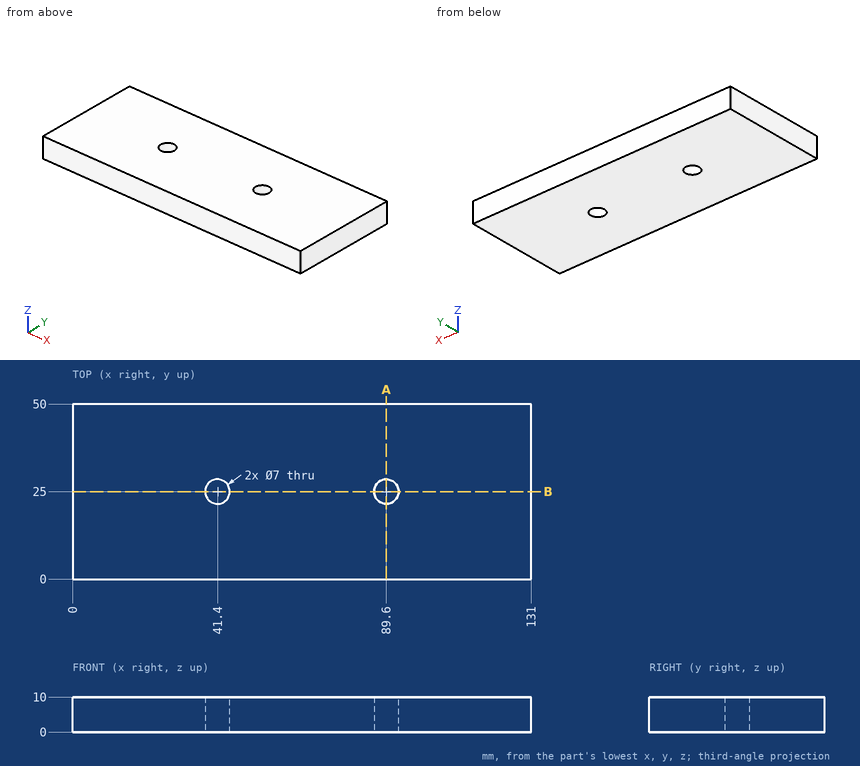
Could you check a few things on this drawing? It's one solid part, dimensions in mm from its lowest x, y, z. Coordinates: 2 decimals unless noted, no trailing zeros. Write each loop counter-clockwise with the first axis right and the second up, starting at its lowest first coordinate (ties: lowest second). Pieces come first, ordered by that corner, then holes. Notation, with made-up numbers: (13, -7.75) - (30, -7.75) arc R9 ccw to (30, 1.25) - close; hole circle Ø9 at (75.25, 21.25). An arc over 180 degrees is marked (long way). Put each result on its own line as item: value. Start each with the question number.
Q1. Please list where these lines run through material, in increasing order: L1, parallel to Y at x = 41.4, z = 6.5; L2, parallel to X at y = 22.5, z = 7.25; L3, parallel to X at y = 28, z = 8.5.
Q2. I want a section at A-A on x = 89.6. Write out the boundary of the cut face in (y, z), plus the area to 3 significant figures.
Q3. I want a section at B-B on y = 25. Write out the boundary of the cut face in (x, z).
Checks:
1. L1: 0 to 21.5, 28.5 to 50
1. L2: 0 to 38.95, 43.85 to 87.15, 92.05 to 131
1. L3: 0 to 39.6, 43.2 to 87.8, 91.4 to 131
2. outline: (0, 0) - (21.5, 0) - (21.5, 10) - (0, 10) - close; (28.5, 0) - (50, 0) - (50, 10) - (28.5, 10) - close
2. area: 430 mm²
3. outline: (0, 0) - (37.9, 0) - (37.9, 10) - (0, 10) - close; (44.9, 0) - (86.1, 0) - (86.1, 10) - (44.9, 10) - close; (93.1, 0) - (131, 0) - (131, 10) - (93.1, 10) - close
